Work out the finished part from the listing and answer in its coordinate system (mm). Round coordinates to 2 decimals unless told otherwise and drop trailing zeros. Order: outer loops, then holes, each group sorted by start corner. A loop starts at its lowest first (then second) coordinate and runs counter-clockwise, first axis right, second up. Notation, with made-up numbers: (32, 81.25) - (90, 81.25) arc R29 ccw to (90, 108.25) - close; hole circle Ø6 at (41, 22). An arc over 180 degrees is marked (long way). Use one line per item in the form item = value. Start each with the question number.
Q1. Find the intervals of material crossed by line 1 (Z direction, x = -3.5, y = -4.25); line 2 (X direction, y = -1.5, z = 13); line 3 (X direction, y = 2.5, z = -30), in increasing order. Write a range as [from, to].
Q2. The part is cut by section C-C on y = -2.5. Determine the outline of the cut face in (x, z), plus the area to 3 significant figures.
Q3. The part is cut by section A-A on z = 27. Determine the outline of the cut face in (x, y), plus the area to 3 significant figures.
Q4. Given P1, Ø1, axis at y = -5, z = 25.5, coming from the -X side, flat-ended and moving along its own axis, determine where the tip first touches the part or whether it passes through.
Q5. The part is cut by section D-D on y = 2.25. Determine the outline of the cut face in (x, z).
Q6. The part is cut by section B-B on x = 6.5. Determine the outline of the cut face in (y, z).
from build123d import *

# Parameters (mm, degrees)
BOSS_EXTRUDE1_DEPTH = 34.13125
SKETCH2_W           = 1.1684
SKETCH2_H           = 4.415483176


with BuildPart() as part:
    # Sketch1 → Boss-Extrude1 (new, symmetric)
    with BuildSketch(Plane.XY):
        Polygon((-3.666174209, 6.35), (-7.332348419, 0), (-3.666174209, -6.35), (3.666174209, -6.35), (7.332348419, 0), (3.666174209, 6.35), align=None)
    extrude(amount=BOSS_EXTRUDE1_DEPTH, both=True)

    # Sketch2 → Cut-Revolve1 (revolve, cut)
    with BuildSketch(Plane(origin=(0, 0, 0), x_dir=(0, 0, -1), z_dir=(1, 0, 0))):
        with Locations((-32.3342, 7.262341588)):
            Rectangle(SKETCH2_W, SKETCH2_H)
    cut_revolve1 = revolve(axis=Axis((0, 0, 0), (0, 0, 1)), mode=Mode.SUBTRACT)

    # Mirror1: Cut-Revolve1 across plane
    add(cut_revolve1.mirror(Plane.XY), mode=Mode.SUBTRACT)


solid = part.part
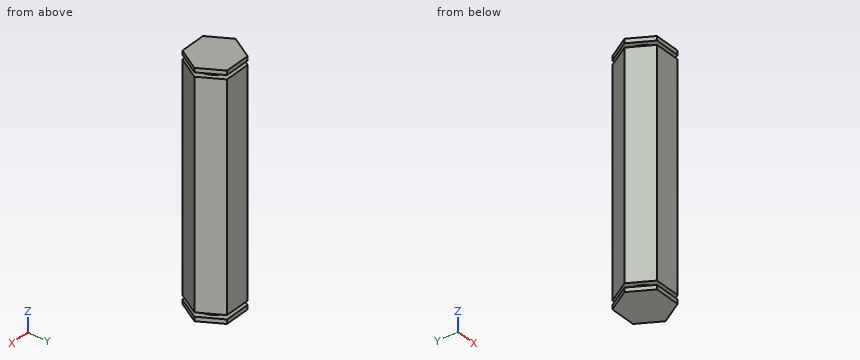
Found:
q1.line_1 = [-34.13, -32.92], [-31.75, 31.75], [32.92, 34.13]
q1.line_2 = [-6.47, 6.47]
q1.line_3 = [-5.89, 5.89]
q2.outline = (-5.89, -34.13) - (5.89, -34.13) - (5.89, -32.92) - (4.39, -32.92) - (4.39, -31.75) - (5.89, -31.75) - (5.89, 31.75) - (4.39, 31.75) - (4.39, 32.92) - (5.89, 32.92) - (5.89, 34.13) - (-5.89, 34.13) - (-5.89, 32.92) - (-4.39, 32.92) - (-4.39, 31.75) - (-5.89, 31.75) - (-5.89, -31.75) - (-4.39, -31.75) - (-4.39, -32.92) - (-5.89, -32.92) - close
q2.area = 797 mm²
q3.outline = (-7.33, 0) - (-3.67, -6.35) - (3.67, -6.35) - (7.33, 0) - (3.67, 6.35) - (-3.67, 6.35) - close
q3.area = 140 mm²
q4.P1 = -4.73
q5.outline = (-6.03, -34.13) - (6.03, -34.13) - (6.03, -32.92) - (4.53, -32.92) - (4.53, -31.75) - (6.03, -31.75) - (6.03, 31.75) - (4.53, 31.75) - (4.53, 32.92) - (6.03, 32.92) - (6.03, 34.13) - (-6.03, 34.13) - (-6.03, 32.92) - (-4.53, 32.92) - (-4.53, 31.75) - (-6.03, 31.75) - (-6.03, -31.75) - (-4.53, -31.75) - (-4.53, -32.92) - (-6.03, -32.92) - close
q6.outline = (-1.44, -34.13) - (1.44, -34.13) - (1.44, -32.92) - (-1.44, -32.92) - close; (-1.44, -31.75) - (1.44, -31.75) - (1.44, 31.75) - (-1.44, 31.75) - close; (-1.44, 32.92) - (1.44, 32.92) - (1.44, 34.13) - (-1.44, 34.13) - close
